```python
from build123d import *

# Parameters (mm, degrees)
SKETCH1_R           = 30
BOSS_EXTRUDE1_DEPTH = 3
BOSS_EXTRUDE2_START = -3
BOSS_EXTRUDE2_DEPTH = 3
SKETCH3_R           = 2.05
CUT_EXTRUDE1_DEPTH  = 105.446158378
CUT_EXTRUDE3_DEPTH  = 105.446158378
FILLET1_R           = 10
FILLET2_R           = 6.5
SKETCH7_R           = 2.55
CUT_EXTRUDE4_DEPTH  = 97.33924434
CIRPATTERN1_COUNT   = 3
SKETCH8_R           = 10
CUT_EXTRUDE5_DEPTH  = 97.33924434


with BuildPart() as part:
    # Sketch1 → Boss-Extrude1 (new body)
    with BuildSketch(Plane(origin=(0, 0, 0), x_dir=(1, 0, 0), z_dir=(0, 1, 0))):
        with Locations(Location((0, 0, 0), (0, 0, 270))):
            Circle(SKETCH1_R)
    extrude(amount=BOSS_EXTRUDE1_DEPTH)

    # Sketch2 → Boss-Extrude2 (add)
    with BuildSketch(Plane(origin=(0, 3, 0), x_dir=(1, 0, 0), z_dir=(0, 1, 0)).offset(BOSS_EXTRUDE2_START)):
        with BuildLine():
            Line((100, 6.5), (29.287369291, 6.5))
            ThreePointArc((29.287369291, 6.5), (25.430321552, 15.915361943), (18.648056199, 23.5))
            Line((18.648056199, 23.5), (100, 23.5))
            Line((100, 23.5), (100, 6.5))
        make_face()
        with BuildLine():
            Line((29.287369291, -6.5), (100, -6.5))
            Line((100, -6.5), (100, -23.5))
            Line((100, -23.5), (18.648056199, -23.5))
            ThreePointArc((18.648056199, -23.5), (25.430321552, -15.915361943), (29.287369291, -6.5))
        make_face()
    extrude(amount=BOSS_EXTRUDE2_DEPTH)

    # Sketch3 → Cut-Extrude1 (cut, through all)
    with BuildSketch(Plane(origin=(0, 3, 0), x_dir=(1, 0, 0), z_dir=(0, 1, 0))):
        with Locations(Location((53, 15, 0), (0, 0, 270))):
            Circle(SKETCH3_R)
        with Locations(Location((83, 15, 0), (0, 0, 270))):
            Circle(SKETCH3_R)
        with Locations(Location((53, -15, 0), (0, 0, 270))):
            Circle(SKETCH3_R)
        with Locations(Location((83, -15, 0), (0, 0, 270))):
            Circle(SKETCH3_R)
    extrude(amount=-CUT_EXTRUDE1_DEPTH, mode=Mode.SUBTRACT)

    # Sketch6 → Cut-Extrude3 (cut, through all)
    with BuildSketch(Plane(origin=(0, 3, 0), x_dir=(1, 0, 0), z_dir=(0, 1, 0))):
        with BuildLine():
            Line((100, 23.5), (83, 23.5))
            ThreePointArc((83, 23.5), (91.5, 15), (83, 6.5))
            Line((83, 6.5), (100, 6.5))
            Line((100, 6.5), (100, 23.5))
        make_face()
        with BuildLine():
            Line((100, -6.5), (83, -6.5))
            ThreePointArc((83, -6.5), (91.5, -15), (83, -23.5))
            Line((83, -23.5), (100, -23.5))
            Line((100, -23.5), (100, -6.5))
        make_face()
    extrude(amount=-CUT_EXTRUDE3_DEPTH, mode=Mode.SUBTRACT)

    # Fillet1
    fillet1_edges = [part.edges().sort_by_distance(p)[0] for p in [
        (18.648056199, 1.5, 23.5),
        (18.648056199, 1.5, -23.5),
    ]]
    fillet(fillet1_edges, radius=FILLET1_R)

    # Fillet2
    fillet2_edges = [part.edges().sort_by_distance(p)[0] for p in [
        (29.287369291, 1.5, 6.5),
        (29.287369291, 1.5, -6.5),
    ]]
    fillet(fillet2_edges, radius=FILLET2_R - 0.0001)  # a hair under: the kernel refuses the full size

    # Sketch7 → Cut-Extrude4 (cut, through all)
    with BuildSketch(Plane(origin=(0, 3, 0), x_dir=(1, 0, 0), z_dir=(0, 1, 0))):
        with Locations(Location((-15.25, 0, 0), (0, 0, 270))):
            Circle(SKETCH7_R)
    cut_extrude4 = extrude(amount=-CUT_EXTRUDE4_DEPTH, mode=Mode.SUBTRACT)

    # CirPattern1: Cut-Extrude4 ×3 about axis
    cirpattern1_axis = Axis((0, 0, 0), (0, 1, 0))
    for i in range(1, CIRPATTERN1_COUNT):
        add(cut_extrude4.rotate(cirpattern1_axis, i * 360 / CIRPATTERN1_COUNT), mode=Mode.SUBTRACT)

    # Sketch8 → Cut-Extrude5 (cut, through all)
    with BuildSketch(Plane(origin=(0, 3, 0), x_dir=(1, 0, 0), z_dir=(0, 1, 0))):
        with Locations(Location((0, 0, 0), (0, 0, 270))):
            Circle(SKETCH8_R)
    extrude(amount=-CUT_EXTRUDE5_DEPTH, mode=Mode.SUBTRACT)


solid = part.part
```
Geometry check sheet. Reference: the model listing, model coordinates, mm. A direction names the side the tool comes from. Give positions to 0.01 mm unless a question says otherwise; leave off trailing zeros. Order: outer loops, then holes, each group sorted by start corner. A loop starts at its lowest first (then second) coordinate and runs counter-clockwise, first axis right, second up. Notation, with made-up numbers: (75.25, -29.5) - (124.25, -29.5) arc R16 ccw to (124.25, -19.5) - close; hole circle Ø6 at (-32, 9.5). An arc over 180 degrees is marked (long way). Write item = value, one per line. Start each with the question number.
1) Scan lines: L1, parallel to X at y = 0.5, z = -14; L2, parallel to X at y = 1.2, z = 0; L3, parallel to X at y = 0.7, z = 16.5. Record each from-to range of solid material in increasing order.
2) Draft check along X on faces 4 (the cylindrical face through (-29.986, 1.479, -0.902)), 5 (the flat face through (32, 0, -7)), 6 (the cylindrical face through (85.033, 1.521, 14.733)), 7 (the cylindrical face through (7.737, 1.521, -15.754)). Enter one of: released by +X, released by -X, zero draft, split by the parting line, or undercut.
3) Section check A-A (x = 53). Enter the section's corners in (y, z), then the cut area to 3 significant figures.
4) Access from +Z, -Z, +X, -X, +Y, -Y to the whole of each face (thin tool, end or side, straight path). Record for faces 1 (the flat face through (52, 1, -23.5)), 2 (the cylindrical face through (31.955, 1.521, 4.646)), 3 (the cylindrical face through (-17.5, 1.5, 1.2)).
5) Gauge pin test, flat ends, axial feed: pin 1 Ø1.5 at (x, y) = (67, 1) entering from +Z; pin 2 Ø4 at (x, z) = (7.62, 13.21) entering from -Y; pin 3 Ø1.5 at (y, z) = (1, 23.5) entering from +X; pin 4 Ø0.9 at (x, y) = (57.5, 1) entering from -Z. Record the tip position at first contact, or that the pin passes through.
6) Section check C-C (x = 78). Enter the section's corners in (y, z).
7) Section check D-D (y = 0.45). Count the separate pieces of the cut face and the enclosed holes in it, then the cut area to 3 significant figures.
8) Section check B-B (z = -4). Enter the section's corners in (x, y), then the cut area to 3 significant figures.
Geometry check:
q1.L1 = -26.53 to 5.2, 10.05 to 51.21, 54.79 to 81.21, 84.79 to 91.44
q1.L2 = -30 to -17.8, -12.7 to -10, 10 to 30
q1.L3 = -25.05 to 51.6, 54.4 to 81.6, 84.4 to 91.37
q2.face_4 = split by the parting line
q2.face_5 = zero draft
q2.face_6 = undercut
q2.face_7 = undercut
q3.outline = (0, -23.5) - (3, -23.5) - (3, -17.05) - (0, -17.05) - close; (0, -12.95) - (3, -12.95) - (3, -6.5) - (0, -6.5) - close; (0, 6.5) - (3, 6.5) - (3, 12.95) - (0, 12.95) - close; (0, 17.05) - (3, 17.05) - (3, 23.5) - (0, 23.5) - close
q3.area = 77.4 mm2
q4.face_1 = -Z, +X, +Y, -Y
q4.face_2 = +X, +Y, -Y
q4.face_3 = +Y, -Y
q5.pin_1 = 23.5
q5.pin_2 = through
q5.pin_3 = 86.49
q5.pin_4 = -23.5
q6.outline = (0, -23.5) - (3, -23.5) - (3, -6.5) - (0, -6.5) - close; (0, 6.5) - (3, 6.5) - (3, 23.5) - (0, 23.5) - close
q7.separate_pieces = 1
q7.enclosed_holes = 8
q7.area = 4,610 mm2
q8.outline = (-29.73, 0) - (-9.17, 0) - (-9.17, 3) - (-29.73, 3) - close; (9.17, 0) - (31.38, 0) - (31.38, 3) - (9.17, 3) - close
q8.area = 128 mm2
